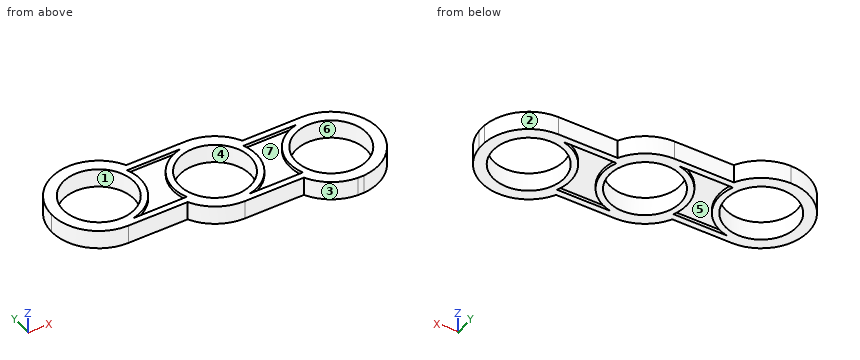
from build123d import *

# Parameters (mm, degrees)
F0_R        = 14.351
F1_DEPTH    = 7.62
F2_T        = 2.54
F2_T3_DEPTH = 12.7
F4_DEPTH    = 7.62
F5_DEPTH    = 1.27
F7_DEPTH    = 1.27


# Not quite as in the source:
# - a shell that OpenCascade refuses in one call is made with other operations: the cavity is built on its own and cut out


with BuildPart() as f1:
    # F0 (on Top) → F1 (new body)
    with BuildSketch(Plane.XY):
        with BuildLine():
            ThreePointArc((-40.64, -9.05), (-27.1696158184, -3.4703841816), (-21.59, 10))
            ThreePointArc((-21.59, 10), (-22.1705835176, 14.6672427406), (-23.8769453858, 19.05))
            ThreePointArc((-23.8769453858, 19.05), (-30.880389352, 26.3600886306), (-40.64, 29.05))
            ThreePointArc((-40.64, 29.05), (-54.0574684375, 23.5230928684), (-59.6894143559, 10.1493743547))
            ThreePointArc((-59.6894143559, 10.1493743547), (-54.1630928684, -3.4174684375), (-40.64, -9.05))
        make_face()
        with Locations((-40.64, 10)):
            Circle(F0_R, mode=Mode.SUBTRACT)
        with BuildLine():
            ThreePointArc((-23.8769453858, 19.05), (-22.1705835176, 14.6672427406), (-21.59, 10))
            ThreePointArc((-21.59, 10), (-27.1696158184, -3.4703841816), (-40.64, -9.05))
            Line((-40.64, -9.05), (-16.7630546142, -9.05))
            ThreePointArc((-16.7630546142, -9.05), (-16.3600886306, 9.759610648), (0, 19.05))
            Line((0, 19.05), (-23.8769453858, 19.05))
        make_face()
        with BuildLine():
            ThreePointArc((16.7630546142, 9.05), (9.759610648, 16.3600886306), (0, 19.05))
            ThreePointArc((0, 19.05), (-16.3600886306, 9.759610648), (-16.7630546142, -9.05))
            ThreePointArc((-16.7630546142, -9.05), (-9.759610648, -16.3600886306), (0, -19.05))
            ThreePointArc((0, -19.05), (13.4703841816, -13.4703841816), (19.05, 0))
            ThreePointArc((19.05, 0), (18.4694164824, 4.6672427406), (16.7630546142, 9.05))
        make_face()
        Circle(F0_R, mode=Mode.SUBTRACT)
        with BuildLine():
            Line((40.64, 9.05), (16.7630546142, 9.05))
            ThreePointArc((16.7630546142, 9.05), (18.4694164824, 4.6672427406), (19.05, 0))
            ThreePointArc((19.05, 0), (13.4703841816, -13.4703841816), (0, -19.05))
            Line((0, -19.05), (23.8769453858, -19.05))
            ThreePointArc((23.8769453858, -19.05), (24.2799113694, -0.240389352), (40.64, 9.05))
        make_face()
        with BuildLine():
            ThreePointArc((59.6056254338, -8.2090360401), (53.4615567808, 4.0893641346), (40.64, 9.05))
            ThreePointArc((40.64, 9.05), (24.2799113694, -0.240389352), (23.8769453858, -19.05))
            ThreePointArc((23.8769453858, -19.05), (30.3891760199, -26.0568710442), (39.4861384834, -29.0150231028))
            Line((39.4861384834, -29.0150231028), (41.7938615166, -29.0150231028))
            ThreePointArc((41.7938615166, -29.0150231028), (53.8825636539, -23.6944152074), (59.6056254338, -11.7909639599))
            Line((59.6056254338, -11.7909639599), (59.6056254338, -8.2090360401))
        make_face()
        with Locations((40.64, -10)):
            Circle(F0_R, mode=Mode.SUBTRACT)
    extrude(amount=F1_DEPTH)

    # F2: shell of thickness 2.54, made by hand


with BuildPart() as f2_core1:
    # F2_t2: copy of F1
    add(f1.part)

    # the walls: a layer under each face that stays
    f2_faces = [f2_core1.faces().sort_by_distance(p)[0] for p in [
        (-57.0000886306, 19.759610648, 3.81),
        (-28.7015273071, -9.05, 3.81),
        (-9.759610648, -16.3600886306, 3.81),
        (11.9384726929, -19.05, 3.81),
        (30.3891760199, -26.0568710442, 3.81),
        (40.64, -29.0150231028, 3.81),
        (53.8825636539, -23.6944152074, 3.81),
        (59.6056254338, -10, 3.81),
        (53.4615567808, 4.0893641346, 3.81),
        (28.7015273071, 9.05, 3.81),
        (9.759610648, 16.3600886306, 3.81),
        (-11.9384726929, 19.05, 3.81),
        (-54.991, 10, 3.81),
        (-14.351, 0, 3.81),
        (26.289, -10, 3.81),
        (-51.1688838976, 0.0174884486, 0),
    ]]
    thicken(f2_faces, amount=-F2_T, mode=Mode.SUBTRACT)

    # F2_s4 → F2_t3 (cut)
    with BuildSketch(Plane.XY.offset(-2.54)):
        Polygon((-23.8545946463, 19.0874666667), (-26.1120193343, 17.8433333333), (-25.3921823509, 16.51), (-23.8769453858, 16.51), align=None)
        Polygon((-16.7854053537, -9.0874666667), (-16.7630546142, -6.51), (-15.2478176491, -6.51), (-14.5279806657, -7.8433333333), align=None)
        Polygon((23.8545946463, -19.0874666667), (23.8769453858, -16.51), (25.3921823509, -16.51), (26.1120193343, -17.8433333333), align=None)
        Polygon((16.7854053537, 9.0874666667), (16.7630546142, 6.51), (15.2478176491, 6.51), (14.5279806657, 7.8433333333), align=None)
    extrude(amount=F2_T3_DEPTH, mode=Mode.SUBTRACT)


with BuildPart() as f1_1:
    add(f1.part)

    # what is left inside the walls is the cavity
    f2_cavity = [f2_core1.part.solids().sort_by_distance(p)[0] for p in [
        (-20.32, 1.163333, 7.5946),
        (20.32, -8.836667, 7.5946),
    ]]
    add(f2_cavity, mode=Mode.SUBTRACT)

    # F3 (on face) → F4 (join)
    with BuildSketch(Plane.XY.offset(7.62)):
        with BuildLine():
            ThreePointArc((-15.5860765108, -6.51), (-14.9730845713, 7.8174560709), (-3.5673212639, 16.51))
            Line((-3.5673212639, 16.51), (-25.0539234892, 16.51))
            ThreePointArc((-25.0539234892, 16.51), (-25.6669154287, 2.1825439291), (-37.0726787361, -6.51))
            Line((-37.0726787361, -6.51), (-15.5860765108, -6.51))
        make_face()
        with BuildLine():
            ThreePointArc((25.0539234892, -16.51), (25.6669154287, -2.1825439291), (37.0726787361, 6.51))
            Line((37.0726787361, 6.51), (15.5860765108, 6.51))
            ThreePointArc((15.5860765108, 6.51), (14.9730845713, -7.8174560709), (3.5673212639, -16.51))
            Line((3.5673212639, -16.51), (25.0539234892, -16.51))
        make_face()
    extrude(amount=-F4_DEPTH)

    # F3 (on face) → F5 (cut)
    with BuildSketch(Plane.XY.offset(7.62)):
        with BuildLine():
            ThreePointArc((-15.5860765108, -6.51), (-14.9730845713, 7.8174560709), (-3.5673212639, 16.51))
            Line((-3.5673212639, 16.51), (-25.0539234892, 16.51))
            ThreePointArc((-25.0539234892, 16.51), (-25.6669154287, 2.1825439291), (-37.0726787361, -6.51))
            Line((-37.0726787361, -6.51), (-15.5860765108, -6.51))
        make_face()
        with BuildLine():
            ThreePointArc((25.0539234892, -16.51), (25.6669154287, -2.1825439291), (37.0726787361, 6.51))
            Line((37.0726787361, 6.51), (15.5860765108, 6.51))
            ThreePointArc((15.5860765108, 6.51), (14.9730845713, -7.8174560709), (3.5673212639, -16.51))
            Line((3.5673212639, -16.51), (25.0539234892, -16.51))
        make_face()
    extrude(amount=-F5_DEPTH, mode=Mode.SUBTRACT)

    # F6 (on face) → F7 (cut)
    with BuildSketch(Plane(origin=(0, 0, 0), x_dir=(1, 0, 0), z_dir=(0, 0, -1))):
        with BuildLine():
            Line((-15.5860765108, 6.51), (-37.0726787361, 6.51))
            ThreePointArc((-37.0726787361, 6.51), (-25.6669154287, -2.1825439291), (-25.0539234892, -16.51))
            Line((-25.0539234892, -16.51), (-3.5673212639, -16.51))
            ThreePointArc((-3.5673212639, -16.51), (-14.9730845713, -7.8174560709), (-15.5860765108, 6.51))
        make_face()
        with BuildLine():
            Line((15.5860765108, -6.51), (37.0726787361, -6.51))
            ThreePointArc((37.0726787361, -6.51), (25.6669154287, 2.1825439291), (25.0539234892, 16.51))
            Line((25.0539234892, 16.51), (3.5673212639, 16.51))
            ThreePointArc((3.5673212639, 16.51), (14.9730845713, 7.8174560709), (15.5860765108, -6.51))
        make_face()
    extrude(amount=-F7_DEPTH, mode=Mode.SUBTRACT)


solid = f1_1.part
Here's how the part is built. I have some questions about the finished solid (model axes, mm). Face numbers are marked on the shaded views. A direction names the side the tool comes from. Give positions to 0.01 mm unless a question says otherwise; leave off trailing zeros. Order: outer loops, then holes, each group sorted by start corner. A loop starts at its lowest first (then second) coordinate and runs counter-clockwise, first axis right, second up. Notation, with made-up numbers: M -34,69.25 L -3,69.25 A33 cw -3,101.25 Z; hole C 40.25,37.5 d10. An arc over 180 degrees is marked long. Answer as a JSON object with one key per item and string values. Group by question number.
1) Please list where these lines run through material, in increasing order: L1, parallel to Y at x = 40.64, z = 6; L2, parallel to X at y = 0.5, z = 2.25. Write a range as [from, to].
2) Suppose I cut it at B-B, the plane z = 3.75. Write out the boundary of the cut face in (x, y).
3) Suppose I cut it at A-A, the plane x = -5. Write out the boundary of the cut face in (y, z).
4) I'm going to push flat-ended pins straight in: pin 1 Ø0.6 at (x, z) = (30, 7) entering from -Y; pin 2 Ø4 at (y, z) = (-6.5, 2.5) entering from -X; pin 3 Ø1 at (x, z) = (25.5, 0.5) entering from -Y; pin 4 Ø4 at (y, z) = (-6.5, 1.5) entering from +X. Where does each tip first touch, or does it pass through?
5) On a 3-axis mill with a long thin cutter (end or side, diameter ignored), from which of +Z, -Z, +X, -X, +Y, -Y can I reach the whole of each face in a straight line? I mean the marked faces 5, 6 and 7. Say none if no direction works.
6) Suppose I cut it at C-C, the plane x = 22. Write out the boundary of the cut face in (y, z), plus the area to 3 significant figures.
7) We'd pull the mould along X, two halves only. Please class the marked faces 1, 2, 3 and 4: pulls with the +X half, pulls with the -X half, needs draft (parallel to the pull), parting line crosses it, or undercut.
8) Suppose I cut it at D-D, the plane x = 49. Write out the boundary of the cut face in (y, z), plus the area to 3 significant figures.
Results found:
{
 "1": {"L1": "[-29.02, -24.35], [4.35, 9.05]", "L2": "[-57.15, -51.4], [-29.88, -14.34], [14.34, 30.86], [50.42, 56.54]"},
 "2": {"outline": "M -40.64,-9.05 L -16.76,-9.05 A19.05 ccw 0,-19.05 L 23.88,-19.05 A19.05 ccw 39.49,-29.02 L 41.79,-29.02 A19.05 ccw 59.61,-11.79 L 59.61,-8.21 A19.05 ccw 40.64,9.05 L 16.76,9.05 A19.05 ccw 0,19.05 L -23.88,19.05 A19.05 ccw long Z; hole C -40.64,10 d28.7; hole C 0,0 d28.7; hole C 40.64,-10 d28.7"},
 "3": {"outline": "M -18.38,0 L -13.45,0 L -13.45,7.62 L -18.38,7.62 Z; M 13.45,0 L 16.13,0 L 16.13,1.27 L 16.51,1.27 L 16.51,0 L 19.05,0 L 19.05,7.62 L 16.51,7.62 L 16.51,6.35 L 16.13,6.35 L 16.13,7.62 L 13.45,7.62 Z"},
 "4": {"pin 1": "y = -26", "pin 2": "x = -53", "pin 3": "y = -22.19", "pin 4": "x = 59.61"},
 "5": {"face 5": "-Z", "face 6": "+Z, -Z", "face 7": "+Z"},
 "6": {"outline": "M -19.05,0 L -16.51,0 L -16.51,1.27 L 6.51,1.27 L 6.51,0 L 9.05,0 L 9.05,7.62 L 6.51,7.62 L 6.51,6.35 L -16.51,6.35 L -16.51,7.62 L -19.05,7.62 Z", "area": "156 mm²"},
 "7": {"face 1": "undercut", "face 2": "pulls with the +X half", "face 3": "pulls with the -X half", "face 4": "undercut"},
 "8": {"outline": "M -27.12,0 L -21.66,0 L -21.66,7.62 L -27.12,7.62 Z; M 1.66,0 L 7.12,0 L 7.12,7.62 L 1.66,7.62 Z", "area": "83.1 mm²"}
}
